The model under review builds one solid part; all positions refer to its coordinate system, in mm. Face numbers are marked on the shaded views. A direction names the side the tool comes from. Coordinates: 2 decimals unless noted, no trailing zeros. Write each loop counter-clockwise with the first axis right and the second up, starting at its lowest first coordinate (ties: lowest second). Pieces come first, ordered by that corner, then holes. Notation, with made-up numbers: (89.5, 74) - (96.5, 74) arc R15 cw to (96.5, 99) - close; hole circle Ø6 at (-0.75, -18.75). An arc over 180 degrees is marked (long way). Put each result on its own line as item: value. Start each with the question number.
Item 1: Consider section B-B on z = 2.65. Give the boundary of the cut face in (x, y), then the cut area to 3 significant figures.
Item 2: To check wall thickness, follow L1, parallel to Y at x = 0, z = 2.7; L2, parallel to Y at x = 0, z = 0.4; L3, parallel to Z at x = 0.5, y = 2.5. State the ranges of each line that lie inside material, in increasing order. Write a range as [from, to].
Item 3: Mouldability with a two-part tool opening along Y and no side actions: class the marked faces 3, 4 and 5 as pulls with the +Y half, pulls with the -Y half, needs draft (parallel to the pull), parting line crosses it, or undercut.
Item 4: Machinability: for the marked faces 1 and 2, which of the approach directions +Z, -Z, +X, -X, +Y, -Y give a long, thin tool a straight path to every point of the face, cutting with its end or side? Answer none if there is none.
Item 5: For pin 1 (1.6 mm diameter, centred on x = -8, y = 0, fed in from +Z); pin 2 (4 mm diameter, centred on x = 0, y = 0, fed in from +Z), all flat-tipped, find the tip position at first contact; note any pin that passes through.
Item 6: Consider section A-A on x = 0. Give the boundary of the cut face in (y, z), then the cut area to 3 significant figures.
Item 7: Consider section C-C on y = 8. Give the boundary of the cut face in (x, z).
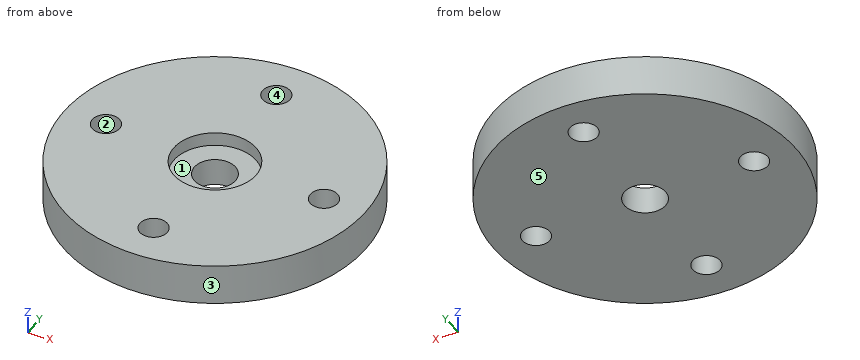
```python
from build123d import *

# Parameters (mm, degrees)
SZKIC1_R                    = 11
SZKIC1_R_2                  = 1
SZKIC1_R_3                  = 1.5
DODANIE_WYCI_GNI_CIE1_DEPTH = 3
SZKIC2_R                    = 3
WYTNIJ_WYCI_GNI_CIE1_DEPTH  = 1


with BuildPart() as part:
    # Szkic1 → Dodanie-wyciągnięcie1 (new body)
    with BuildSketch(Plane.XY):
        Circle(SZKIC1_R)
        with Locations((0, 8)):
            Circle(SZKIC1_R_2, mode=Mode.SUBTRACT)
        with Locations((8, 0)):
            Circle(SZKIC1_R_2, mode=Mode.SUBTRACT)
        with Locations((0, -8)):
            Circle(SZKIC1_R_2, mode=Mode.SUBTRACT)
        with Locations((-8, 0)):
            Circle(SZKIC1_R_2, mode=Mode.SUBTRACT)
        Circle(SZKIC1_R_3, mode=Mode.SUBTRACT)
    extrude(amount=DODANIE_WYCI_GNI_CIE1_DEPTH)

    # Szkic2 → Wytnij-wyciągnięcie1 (cut)
    with BuildSketch(Plane.XY.offset(3)):
        Circle(SZKIC2_R)
    extrude(amount=-WYTNIJ_WYCI_GNI_CIE1_DEPTH, mode=Mode.SUBTRACT)


solid = part.part
```
Report:
1. outline: circle Ø22 at (0, 0); hole circle Ø2 at (-8, 0); hole circle Ø6 at (0, 0); hole circle Ø2 at (0, -8); hole circle Ø2 at (0, 8); hole circle Ø2 at (8, 0)
1. area: 339 mm²
2. L1: [-11, -9], [-7, -3], [3, 7], [9, 11]
2. L2: [-11, -9], [-7, -1.5], [1.5, 7], [9, 11]
2. L3: [0, 2]
3. face 3: parting line crosses it
3. face 4: undercut
3. face 5: needs draft
4. face 1: +Z
4. face 2: +Z, -Z
5. pin 1: through
5. pin 2: z = 2
6. outline: (-11, 0) - (-9, 0) - (-9, 3) - (-11, 3) - close; (-7, 0) - (-1.5, 0) - (-1.5, 2) - (-3, 2) - (-3, 3) - (-7, 3) - close; (1.5, 0) - (7, 0) - (7, 3) - (3, 3) - (3, 2) - (1.5, 2) - close; (9, 0) - (11, 0) - (11, 3) - (9, 3) - close
6. area: 42.0 mm²
7. outline: (-7.55, 0) - (-1, 0) - (-1, 3) - (-7.55, 3) - close; (1, 0) - (7.55, 0) - (7.55, 3) - (1, 3) - close
